from build123d import *

# Parameters (mm, degrees)
BOSS_EXTRUDE2_DEPTH = 127


with BuildPart() as part:
    # Sketch1 → Boss-Extrude2 (new body)
    with BuildSketch(Plane.XY):
        with BuildLine():
            Line((-58.272673139, -67.137959198), (-58.272673139, -519.346809046))
            Line((-58.272673139, -519.346809046), (-336.974932069, -519.346809046))
            Line((-336.974932069, -519.346809046), (-336.974932069, -609.62196559))
            Line((-336.974932069, -609.62196559), (-58.272673139, -609.62196559))
            Line((-58.272673139, -609.62196559), (-58.272673139, -1403.11866405))
            Line((-58.272673139, -1403.11866405), (-84.73010294, -1826.874477175))
            Line((-84.73010294, -1826.874477175), (-53.889938316, -1828.8))
            Line((-53.889938316, -1828.8), (0, -965.671011219))
            Line((0, -965.671011219), (53.889938316, -1828.8))
            Line((53.889938316, -1828.8), (84.73010294, -1826.874477175))
            Line((84.73010294, -1826.874477175), (58.272673139, -1403.11866405))
            Line((58.272673139, -1403.11866405), (58.272673139, -609.62196559))
            Line((58.272673139, -609.62196559), (336.974932069, -609.62196559))
            Line((336.974932069, -609.62196559), (336.974932069, -519.346809046))
            Line((336.974932069, -519.346809046), (58.272673139, -519.346809046))
            Line((58.272673139, -519.346809046), (58.272673139, -67.137959198))
            ThreePointArc((58.272673139, -67.137959198), (0, 88.9), (-58.272673139, -67.137959198))
        make_face()
    extrude(amount=BOSS_EXTRUDE2_DEPTH)


solid = part.part
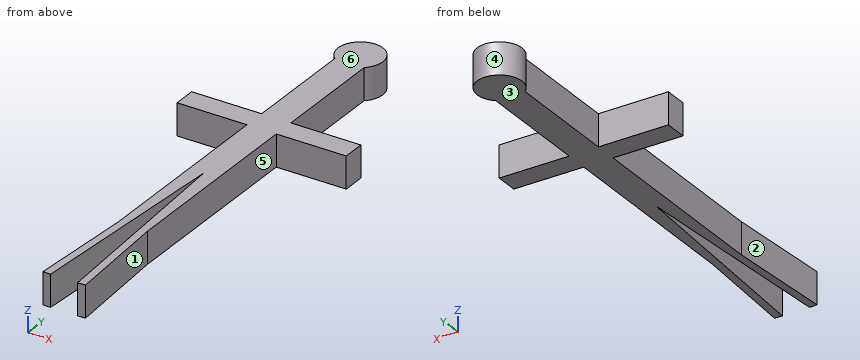
Geometry: final body of the model. Coordinates: model frame, mm. Face numbers are marked on the shaded views. A direction names the side the tool comes from. Give positions to 0.01 mm unless a question says otherwise; leave off trailing zeros. Loops run counter-clockwise (first coordinate to the right, second up) from the corner with the lowest first, then second, coordinate; pieces in that order, holes last. Notation, with made-up numbers: (80.5, 18) - (86.5, 18) arc R21 ccw to (86.5, 31) - close; hole circle Ø4 at (-38, 39). An arc over 180 degrees is marked (long way). One line per question, with ' | ' between items. Start each with the question number.
(1) Pull-direction query (Y, two-part tool) for the marked faces 4, 5 and 6; classes: released by +Y, released by -Y, zero draft, split by the parting line, or undercut.
(2) Section query A-A on z = 65.5. Return loops of the section in (x, y), then the cut area to 3 significant figures.
(3) Reachability of the marked faces 1, 2 and 3 from +Z, -Z, +X, -X, +Y, -Y: full face, straight path, thin tool, end or side. Return the list, or none.
(4) Section query C-C on y = 0. Return loops of the section in (x, z).
(5) Ray query, line 1 (X direction, y = -992.5, z = 78.5); line 2 (X direction, y = -1136, z = 47); line 3 (Y direction, x = -221, z = 86). Return the intervals inside material, ascending. Write a range as from..to.
(6) Section query D-D on x = 286. Return loops of the section in (y, z), then the cut area to 3 significant figures.
(7) Contact query for flat-ended pins moving along their axis: pin 1 (1.5 mm diameter, centred on x = -176, z = 30, fed in from +Y); pin 2 (4 mm diameter, centred on y = -693.5, z = 49, fed in from +X); pin 3 (1 mm diameter, centred on y = -503.5, z = 59.5, fed in from -X). Output: stop coordinate, or through.
(8) Section query B-B on y = -1156. Return loops of the section in (x, z).
The answers:
1) face 4: undercut | face 5: undercut | face 6: zero draft
2) outline: (-336.97, -609.62) - (-58.27, -609.62) - (-58.27, -1403.12) - (-84.73, -1826.87) - (-53.89, -1828.8) - (0, -965.67) - (53.89, -1828.8) - (84.73, -1826.87) - (58.27, -1403.12) - (58.27, -609.62) - (336.97, -609.62) - (336.97, -519.35) - (58.27, -519.35) - (58.27, -67.14) arc R88.9 ccw (long way) to (-58.27, -67.14) - (-58.27, -519.35) - (-336.97, -519.35) - close | area: 243,000 mm2
3) face 1: +Z, -Z, +X | face 2: +Z, -Z, -X | face 3: -Z, +X, -X, +Y, -Y
4) outline: (-88.9, 0) - (88.9, 0) - (88.9, 127) - (-88.9, 127) - close
5) line 1: -58.27..-1.68, 1.68..58.27 | line 2: -58.27..-10.63, 10.63..58.27 | line 3: -609.62..-519.35
6) outline: (-609.62, 0) - (-519.35, 0) - (-519.35, 127) - (-609.62, 127) - close | area: 11,500 mm2
7) pin 1: y = -519.35 | pin 2: x = 58.27 | pin 3: x = -58.27
8) outline: (-58.27, 0) - (-11.88, 0) - (-11.88, 127) - (-58.27, 127) - close; (11.88, 0) - (58.27, 0) - (58.27, 127) - (11.88, 127) - close
